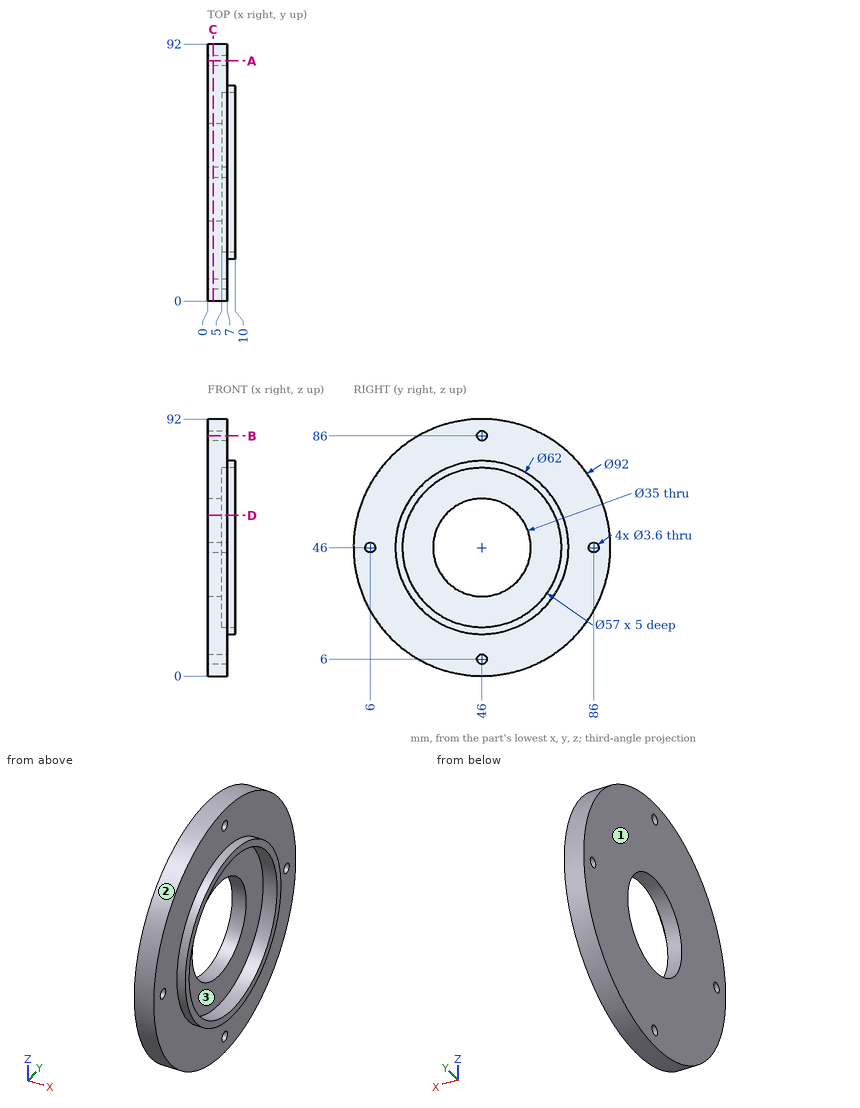
Job drawing, mm, ordinate dimensions from the low corner. One solid piece. Round coordinates to 2 decimals unless told otherwise and drop trailing zeros. Loops run counter-clockwise (first coordinate to the right, second up) from the corner with the lowest first, then second, coordinate; pieces in that order, holes last.
Item 1: Drill centre lines: line 1 (Y direction, x = 3.5, z = 46); line 2 (X direction, y = 71, z = 13); line 3 (Y direction, x = 7.4, z = 46). Where is each one in solid material? Low to high.
Item 2: Cut at C-C, the plane x = 2. Give the cut face in (y, z), then the cut area to 3 significant figures.
Item 3: Drop flat-ended pins along their axis: P1, Ø3, axis at x = 3.5, z = 46, coming from the +Y side; P2, Ø4, axis at y = 46, z = 86, coming from the +X side; P3, Ø2, axis at x = 3.5, z = 58, coming from the -Y side. Give the stop position or say it passes through.
Item 4: Mould opens along Z. For the marked faces 1, 2 and 3 say: +Z half, -Z half, draft (parallel to the pull), parting line (faces both ways), or undercut.
Item 5: Cut at A-A, the plane y = 86. Give the cut face in (x, z), then the cut area to 3 significant figures.
Item 6: Cut at D-D, the plane z = 57.5. Give the cut face in (x, y), then the cut area to 3 significant figures.
A:
1. line 1: y = 0 to 4.2, 7.8 to 28.5, 63.5 to 84.2, 87.8 to 92
1. line 2: x = 0 to 7
1. line 3: y = 15 to 17.5, 74.5 to 77
2. outline: circle Ø92 at (46, 46); hole circle Ø3.6 at (6, 46); hole circle Ø35 at (46, 46); hole circle Ø3.6 at (46, 6); hole circle Ø3.6 at (46, 86); hole circle Ø3.6 at (86, 46)
2. area: 5,640 mm2
3. P1: stops at y = 92
3. P2: stops at x = 7
3. P3: stops at y = 1.33
4. face 1: draft
4. face 2: parting line
4. face 3: undercut
5. outline: (0, 23.28) - (7, 23.28) - (7, 44.2) - (0, 44.2) - close; (0, 47.8) - (7, 47.8) - (7, 68.72) - (0, 68.72) - close
5. area: 293 mm2
6. outline: (0, 1.46) - (7, 1.46) - (7, 17.21) - (10, 17.21) - (10, 19.92) - (5, 19.92) - (5, 32.81) - (0, 32.81) - close; (0, 59.19) - (5, 59.19) - (5, 72.08) - (10, 72.08) - (10, 74.79) - (7, 74.79) - (7, 90.54) - (0, 90.54) - close
6. area: 404 mm2
